The model under review builds one solid part; all positions refer to its coordinate system, in mm. Give positions to 0.01 mm unless a question says otherwise; leave off trailing zeros. Loops run counter-clockwise (first coordinate to the right, second up) from the corner with the lowest first, then second, coordinate; pieces in that order, holes last. Notation, with made-up numbers: M 15,5.25 L 54,5.25 A7 cw 54,15.25 Z; hole C -31.75,39.5 d10. An arc over 180 degrees is marked long. One line per item, written item: value. Start each with the question number.
Q1. We need section A-A on x = 29.5. Write out the cut boundary in (y, z), plus the area to 3 significant figures.
Q2. We need section D-D on x = 48.5. Write out the cut boundary in (y, z).
Q3. We need section C-C on y = 2.75. Give the number of separate pieces and of enclosed holes in the cut face, plus the area to 3 significant figures.
Q4. To check wall thickness, follow line 1 along X through (y, z) = (2.5, 96.1); line 2 along X through (y, z) = (1.5, -25.35); line 3 along Z through (x, y) = (17.85, 2.3). State the ranges of each line that lie inside material, in increasing order. Write a range as from..to.
Q5. For pin 1 (1.2 mm diameter, centred on y = 2, z = 83, fed in from -X), flat-tipped, find the tip position at first contact; note if it passes through.
Q6. We need section B-B on z = -25.35. Write out the cut boundary in (x, y), plus the area to 3 significant figures.
```python
from build123d import *

# Parameters (mm, degrees)
SKETCH1_W           = 75.7
SKETCH1_H           = 42.7
SKETCH1_R           = 1.75
BOSS_EXTRUDE1_DEPTH = 4
SKETCH3_W           = 75.7
SKETCH3_H           = 29.75
SKETCH3_R           = 1.75
BOSS_EXTRUDE2_DEPTH = 4
SKETCH3_3_R         = 1.75
CUT_EXTRUDE1_DEPTH  = 4
SKETCH4_W           = 75.7
SKETCH4_H           = 50
SKETCH4_R           = 1.75
BOSS_EXTRUDE3_DEPTH = 4
SKETCH6_W           = 9
SKETCH6_H           = 8
BOSS_EXTRUDE4_DEPTH = 4
SKETCH6_3_R         = 1.75
CUT_EXTRUDE2_DEPTH  = 115.220007004
SKETCH7_W           = 15.15
SKETCH7_H           = 10
SKETCH7_R           = 1.75
BOSS_EXTRUDE5_DEPTH = 4
SKETCH8_W           = 75.7
SKETCH8_H           = 22
BOSS_EXTRUDE6_DEPTH = 4
SKETCH9_R           = 1.75
CUT_EXTRUDE3_DEPTH  = 135.08433913
BOSS_EXTRUDE7_DEPTH = 4


with BuildPart() as part:
    # Sketch1 → Boss-Extrude1 (new body)
    with BuildSketch(Plane(origin=(0, 0, 0), x_dir=(1, 0, 0), z_dir=(0, 1, 0))):
        Rectangle(SKETCH1_W, SKETCH1_H)
        with Locations(Location((2.4, 17.25, 0), (0, 0, 270))):
            Circle(SKETCH1_R, mode=Mode.SUBTRACT)
        with Locations(Location((-33.8, -17.05, 0), (0, 0, 270))):
            Circle(SKETCH1_R, mode=Mode.SUBTRACT)
        with Locations(Location((29.5, -17.05, 0), (0, 0, 270))):
            Circle(SKETCH1_R, mode=Mode.SUBTRACT)
        with Locations(Location((33.9, 17.25, 0), (0, 0, 270))):
            Circle(SKETCH1_R, mode=Mode.SUBTRACT)
    extrude(amount=BOSS_EXTRUDE1_DEPTH)

    # Sketch3 → Boss-Extrude2 (add)
    with BuildSketch(Plane(origin=(0, 4, 0), x_dir=(1, 0, 0), z_dir=(0, 1, 0))):
        with Locations((0, -36.225)):
            Rectangle(SKETCH3_W, SKETCH3_H)
        with Locations(Location((0, -42.2, 0), (0, 0, 270))):
            Circle(SKETCH3_R, mode=Mode.SUBTRACT)
        with Locations(Location((0, -27.2, 0), (0, 0, 270))):
            Circle(SKETCH3_R, mode=Mode.SUBTRACT)
    extrude(amount=-BOSS_EXTRUDE2_DEPTH)

    # Sketch3<3> → Cut-Extrude1 (cut)
    with BuildSketch(Plane(origin=(0, 4, 0), x_dir=(1, 0, 0), z_dir=(0, 1, 0))):
        with Locations(Location((0, 5.6, 0), (0, 0, 270))):
            Circle(SKETCH3_3_R)
        with Locations(Location((0, -9.4, 0), (0, 0, 270))):
            Circle(SKETCH3_3_R)
    extrude(amount=-CUT_EXTRUDE1_DEPTH, mode=Mode.SUBTRACT)

    # Sketch4 → Boss-Extrude3 (add)
    # profile 1 of 2: a face of its own
    with BuildSketch(Plane(origin=(0, 0, 0), x_dir=(1, 0, 0), z_dir=(0, 1, 0))):
        with Locations((0, -76.1)):
            Rectangle(SKETCH4_W, SKETCH4_H)
        with Locations(Location((-32.85, -56.1, 0), (0, 0, 270))):
            Circle(SKETCH4_R, mode=Mode.SUBTRACT)
        with Locations(Location((-17.85, -56.1, 0), (0, 0, 270))):
            Circle(SKETCH4_R, mode=Mode.SUBTRACT)
        with Locations(Location((-17.85, -96.1, 0), (0, 0, 270))):
            Circle(SKETCH4_R, mode=Mode.SUBTRACT)
        with Locations(Location((-32.85, -96.1, 0), (0, 0, 270))):
            Circle(SKETCH4_R, mode=Mode.SUBTRACT)
        with Locations(Location((32.85, -96.1, 0), (0, 0, 90))):
            Circle(SKETCH4_R, mode=Mode.SUBTRACT)
        with Locations(Location((17.85, -96.1, 0), (0, 0, 90))):
            Circle(SKETCH4_R, mode=Mode.SUBTRACT)
        with Locations(Location((17.85, -56.1, 0), (0, 0, 90))):
            Circle(SKETCH4_R, mode=Mode.SUBTRACT)
        with Locations(Location((32.85, -56.1, 0), (0, 0, 90))):
            Circle(SKETCH4_R, mode=Mode.SUBTRACT)
    # profile 2 of 2: a face of its own
    with BuildSketch(Plane(origin=(0, 0, 0), x_dir=(1, 0, 0), z_dir=(0, 1, 0))):
        Polygon((-37.85, 21.35), (-44, 21.35), (-44, 29.35), (44, 29.35), (44, 21.35), (37.85, 21.35), align=None)
    extrude(amount=BOSS_EXTRUDE3_DEPTH)

    # Sketch6 → Boss-Extrude4 (add)
    with BuildSketch(Plane(origin=(0, 4, 0), x_dir=(1, 0, 0), z_dir=(0, 1, 0))):
        with Locations((-48.5, 25.35)):
            Rectangle(SKETCH6_W, SKETCH6_H)
        with Locations((48.5, 25.35)):
            Rectangle(SKETCH6_W, SKETCH6_H)
    extrude(amount=-BOSS_EXTRUDE4_DEPTH)

    # Sketch6<3> → Cut-Extrude2 (cut, through all)
    with BuildSketch(Plane(origin=(0, 4, 0), x_dir=(1, 0, 0), z_dir=(0, 1, 0))):
        with Locations(Location((0, 25.35, 0), (0, 0, 270))):
            Circle(SKETCH6_3_R)
        with Locations(Location((20.5, 25.35, 0), (0, 0, 270))):
            Circle(SKETCH6_3_R)
        with Locations(Location((41, 25.35, 0), (0, 0, 270))):
            Circle(SKETCH6_3_R)
        with Locations(Location((-20.5, 25.35, 0), (0, 0, 270))):
            Circle(SKETCH6_3_R)
        with Locations(Location((-41, 25.35, 0), (0, 0, 270))):
            Circle(SKETCH6_3_R)
    extrude(amount=-CUT_EXTRUDE2_DEPTH, mode=Mode.SUBTRACT)

    # Sketch7 → Boss-Extrude5 (add)
    # profile 1 of 2: a face of its own
    with BuildSketch(Plane(origin=(0, 0, 0), x_dir=(1, 0, 0), z_dir=(0, 1, 0))):
        with Locations((-45.425, 16.35)):
            Rectangle(SKETCH7_W, SKETCH7_H)
        with Locations(Location((-48.5, 16.35, 0), (0, 0, 270))):
            Circle(SKETCH7_R, mode=Mode.SUBTRACT)
    # profile 2 of 2: a face of its own
    with BuildSketch(Plane(origin=(0, 0, 0), x_dir=(1, 0, 0), z_dir=(0, 1, 0))):
        with Locations((45.425, 16.35)):
            Rectangle(SKETCH7_W, SKETCH7_H)
        with Locations(Location((48.5, 16.35, 0), (0, 0, 270))):
            Circle(SKETCH7_R, mode=Mode.SUBTRACT)
    extrude(amount=BOSS_EXTRUDE5_DEPTH)

    # Sketch8 → Boss-Extrude6 (add)
    with BuildSketch(Plane(origin=(0, 0, 0), x_dir=(1, 0, 0), z_dir=(0, 1, 0))):
        with Locations((0, -112.1)):
            Rectangle(SKETCH8_W, SKETCH8_H)
    extrude(amount=BOSS_EXTRUDE6_DEPTH)

    # Sketch9 → Cut-Extrude3 (cut, through all)
    with BuildSketch(Plane(origin=(0, 4, 0), x_dir=(1, 0, 0), z_dir=(0, 1, 0))):
        with Locations(Location((-12.85, -119.1, 0), (0, 0, 270))):
            Circle(SKETCH9_R)
        with Locations(Location((-32.85, -119.1, 0), (0, 0, 270))):
            Circle(SKETCH9_R)
    cut_extrude3 = extrude(amount=-CUT_EXTRUDE3_DEPTH, mode=Mode.SUBTRACT)

    # Mirror1: Cut-Extrude3 across plane
    add(cut_extrude3.mirror(Plane(origin=(0, 0, 0), x_dir=(0, 0, 1), z_dir=(1, 0, 0))), mode=Mode.SUBTRACT)

    # Sketch10 → Boss-Extrude7 (add)
    with BuildSketch(Plane(origin=(0, 4, 0), x_dir=(1, 0, 0), z_dir=(0, 1, 0))):
        Polygon((-53, 11.35), (-37.85, -43.65), (-37.85, 11.35), align=None)
        Polygon((53, 11.35), (37.85, -43.65), (37.85, 11.35), align=None)
    extrude(amount=-BOSS_EXTRUDE7_DEPTH)


solid = part.part
```
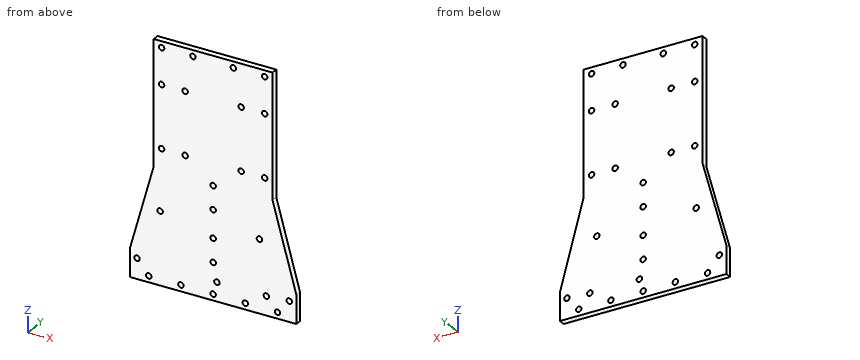
Solved:
1. outline: M 0,-29.35 L 4,-29.35 L 4,15.3 L 0,15.3 Z; M 0,18.8 L 4,18.8 L 4,123.1 L 0,123.1 Z
1. area: 596 mm2
2. outline: M 0,-29.35 L 4,-29.35 L 4,-18.1 L 0,-18.1 Z; M 0,-14.6 L 4,-14.6 L 4,4.99 L 0,4.99 Z
3. separate pieces: 1
3. enclosed holes: 27
3. area: 12,700 mm2
4. line 1: -37.85..-34.6, -31.1..-19.6, -16.1..16.1, 19.6..31.1, 34.6..37.85
4. line 2: -53..-42.75, -39.25..-22.25, -18.75..-1.75, 1.75..18.75, 22.25..39.25, 42.75..53
4. line 3: -29.35..54.35, 57.85..94.35, 97.85..123.1
5. pin 1: x = -37.85
6. outline: M -53,0 L -42.75,0 L -42.75,4 L -53,4 Z; M -39.25,0 L -22.25,0 L -22.25,4 L -39.25,4 Z; M -18.75,0 L -1.75,0 L -1.75,4 L -18.75,4 Z; M 1.75,0 L 18.75,0 L 18.75,4 L 1.75,4 Z; M 22.25,0 L 39.25,0 L 39.25,4 L 22.25,4 Z; M 42.75,0 L 53,0 L 53,4 L 42.75,4 Z
6. area: 354 mm2
